Here's how the part is built. I have some questions about the finished solid (model axes, mm). Give positions to 0.01 mm unless a question says otherwise; leave off trailing zeros. Order: outer loops, then holes, each group sorted by start corner. A loop starts at its lowest first (then second) coordinate and runs counter-clockwise, first axis right, second up.
from build123d import *

# Parameters (mm, degrees)
F0_R     = 4
F0_R_2   = 12.5
F0_R_3   = 5
F1_DEPTH = 10
F3_DEPTH = 10
F5_DEPTH = 10


with BuildPart() as f1:
    # F0 (on Top) → F1 (new body, symmetric)
    with BuildSketch(Plane.XY):
        with BuildLine():
            Line((-20.543962, 242.302258), (-19.634877, -57.696364))
            ThreePointArc((-19.634877, -57.696364), (8.59643, -79.952697), (29.853362, -50.961424))
            Line((29.853362, -50.961424), (-20.543962, 242.302258))
        make_face()
        with BuildLine():
            Line((12.65154, -32.619782), (-6.725958, -32.619782))
            ThreePointArc((-6.725958, -32.619782), (-10.256131, -31.160668), (-11.725935, -27.634933))
            Line((-11.725935, -27.634933), (-11.84751, 12.484849))
            ThreePointArc((-11.84751, 12.484849), (-10.38842, 16.030173), (-6.847533, 17.5))
            Line((-6.847533, 17.5), (5.756961, 17.5))
            ThreePointArc((5.756961, 17.5), (8.979214, 16.32323), (10.684726, 13.346836))
            Line((10.684726, 13.346836), (17.579305, -26.772946))
            ThreePointArc((17.579305, -26.772946), (16.47477, -30.842034), (12.65154, -32.619782))
        make_face(mode=Mode.SUBTRACT)
        with Locations((-4.908372, 32.579835)):
            Circle(F0_R, mode=Mode.SUBTRACT)
        with Locations((-4.999281, 62.579835)):
            Circle(F0_R, mode=Mode.SUBTRACT)
        with Locations((5.226905, -55.193478)):
            Circle(F0_R_2, mode=Mode.SUBTRACT)
        with Locations((-10.44188, 125.224027)):
            Circle(F0_R_3, mode=Mode.SUBTRACT)
        with BuildLine():
            Line((-2.713003, 77.5), (-10.050577, 77.5))
            ThreePointArc((-10.050577, 77.5), (-11.462646, 78.083645), (-12.050567, 79.493939))
            Line((-12.050567, 79.493939), (-12.117614, 101.619189))
            ThreePointArc((-12.117614, 101.619189), (-11.533977, 103.037319), (-10.117623, 103.62525))
            Line((-10.117623, 103.62525), (-6.515225, 103.62525))
            ThreePointArc((-6.515225, 103.62525), (-5.226324, 103.154542), (-4.544118, 101.963984))
            Line((-4.544118, 101.963984), (-0.741897, 79.838734))
            ThreePointArc((-0.741897, 79.838734), (-1.183711, 78.211099), (-2.713003, 77.5))
        make_face(mode=Mode.SUBTRACT)
    extrude(amount=F1_DEPTH, both=True)

    # F2 (on Top) → F3 (join)
    with BuildSketch(Plane.XY):
        with BuildLine():
            Line((-17.758185, 116.28598), (-12.327851, 113.452759))
            Line((-12.327851, 113.452759), (-12.327851, -47.830094))
            ThreePointArc((-12.327851, -47.830094), (1.176909, -74.372973), (23.646388, -54.8275))
            Line((23.646388, -54.8275), (-7.25136, 142.539755))
            Line((-7.25136, 142.539755), (-12.327851, 142.539755))
            Line((-12.327851, 142.539755), (-17.758185, 116.28598))
        make_face()
    extrude(amount=F3_DEPTH)

    # F4 (on Top) → F5 (join)
    with BuildSketch(Plane.XY):
        with BuildLine():
            ThreePointArc((29.503305, -46.357701), (0.523158, -29.868779), (-20.85342, -55.457358))
            ThreePointArc((-20.85342, -55.457358), (4.926275, -81.453466), (31.142796, -55.897952))
            Line((31.142796, -55.897952), (29.503305, -46.357701))
        make_face()
        with BuildLine():
            Line((-20.887821, 246.869915), (-20.85342, -55.457358))
            ThreePointArc((-20.85342, -55.457358), (0.523158, -29.868779), (29.503305, -46.357701))
            Line((29.503305, -46.357701), (-20.887821, 246.869915))
        make_face()
        with BuildLine():
            Line((29.503305, -46.357701), (31.142796, -55.897952))
            ThreePointArc((31.142796, -55.897952), (31.145634, -55.676184), (31.14658, -55.454399))
            ThreePointArc((31.14658, -55.454399), (30.732463, -50.832434), (29.503305, -46.357701))
        make_face()
    extrude(amount=F5_DEPTH)


solid = f1.part
Q1. If we section it at A-A on z = -6: List the corners of the cut face in (x, y) for me, plus the area to 3 significant figures.
Filled sheet:
outline: (-20.54, 242.3) - (-19.63, -57.7) arc R24.99 ccw (long way) to (29.85, -50.96) - close; hole circle Ø10 at (-10.44, 125.22); hole (-12.12, 101.62) - (-12.05, 79.49) arc R2 ccw to (-10.05, 77.5) - (-2.71, 77.5) arc R2 ccw to (-0.74, 79.84) - (-4.54, 101.96) arc R2 ccw to (-6.52, 103.63) - (-10.12, 103.63) arc R2 ccw to start; hole (-11.85, 12.48) - (-11.73, -27.63) arc R5 ccw to (-6.73, -32.62) - (12.65, -32.62) arc R5 ccw to (17.58, -26.77) - (10.68, 13.35) arc R5 ccw to (5.76, 17.5) - (-6.85, 17.5) arc R5 ccw to start; hole circle Ø8 at (-5, 62.58); hole circle Ø8 at (-4.91, 32.58); hole circle Ø25 at (5.23, -55.19)
area: 6,250 mm2
Q2. I need wall thicknesses on L1, parallel to X at y = -53, z = -2; L2, parallel to X at y = 126, z = -1.5; L3, parallel to X at y = 53, z = 1.75. Which ranges of each line are inside material? Lowest first, please.
Filled sheet:
L1: x = -19.65 to -7.08, 17.53 to 30.12
L2: x = -20.19 to -15.38, -5.5 to -0.56
L3: x = -20.87 to 12.43
Q3. I'm going to push flat-ended pins straight in: P1, Ø6, axis at y = 23.5, z = -6, coming from the -X side; P2, Ø8, axis at x = 0, z = -6, coming from the -Y side; P3, Ø1.8, axis at x = -7.5, z = -3.5, coming from the -Y side. Where does each tip first touch, or does it pass through?
Filled sheet:
P1: stops at x = -19.89
P2: stops at y = -80.15
P3: stops at y = -77.2
Q4. If we section it at C-C on z = 6.5: List the corners of the cut face in (x, y) for me, plus the area to 3 significant figures.
Filled sheet:
outline: (-20.89, 246.87) - (-20.85, -55.46) arc R26 ccw to (31.14, -55.9) arc R26 ccw to (31.15, -55.45) arc R26 ccw to (29.5, -46.36) - close
area: 8,910 mm2
Q5. If we section it at B-B on y = 93: List the corners of the cut face in (x, z) for me.
Filled sheet:
outline: (-20.87, 0) - (-20.09, 0) - (-20.09, -10) - (-12.09, -10) - (-12.09, 0) - (-3, 0) - (-3, -10) - (5.11, -10) - (5.11, 0) - (5.55, 0) - (5.55, 10) - (-20.87, 10) - close
Q6. If we section it at D-D on y = 212.5: List the corners of the cut face in (x, z) for me.
Filled sheet:
outline: (-20.88, 0) - (-20.45, 0) - (-20.45, -10) - (-15.42, -10) - (-15.42, 0) - (-14.98, 0) - (-14.98, 10) - (-20.88, 10) - close
Q7. Thinking about a two-plate mould opening in Y: for faces 1 (the face through (-1, 17.5, -5)), 2 (the face through (5.007, 93.618, -4.93)), which applies, released by +Y, released by -Y, zero draft, split by the parting line, or undercut?
Filled sheet:
face 1: undercut
face 2: released by +Y
